Geometry: final body of the model. Coordinates: model frame, mm. Give positions to 0.01 mm unless a question says otherwise; leave off trailing zeros. Order: outer loops, then holes, each group sorted by start corner. A loop starts at its lowest first (then second) coordinate and runs counter-clockwise, first axis right, second up. Notation, with made-up numbers: (22.25, -28) - (70.25, -28) arc R15 ccw to (70.25, -17) - close; hole circle Ø2 at (-28.5, 65). An arc over 180 degrees is marked (long way). Put each result on its own line as item: value. Start each with the question number.
1. Mould query, pull axis X, two halves, no side actions, for faces 1 (the flat face through (30, 30, -8.5)), 2 (the cylindrical face through (48.94, -43.68, -9.01)), 3 (the cylindrical face through (-55.55, -42.594, -8.993)). Classes: pulls with the +X half, pulls with the -X half, needs draft (parallel to the pull), parting line crosses it, or undercut.
2. Section B-B on x = 0. Return the cut outline in (y, z).
3. Section C-C on y = -22. Return the cut outline in (x, z), plus the area to 3 significant figures.
4. Ray query, line 1 along Y through (x, z) = (-6.5, -9.05); line 2 along Y through (x, z) = (41, -8.7); line 3 along Y through (x, z) = (-36.5, -9.1). Return the intervals inside material, ascending. Write a range as from..to.
5. Section D-D on x = 65. Return the cut outline in (y, z), plus the area to 3 significant figures.
6. First-contact query: P1, Ø2.5, axis at x = 42.51, y = 26.32, coming from the -Z side. Flat tip, straight axial feed; report the tip coordinate or a pass-through.
7. Section A-A on y = 0. Return the cut outline in (x, z) (3 decimals), plus the area to 4 significant figures.
from build123d import *

# Parameters (mm, degrees)
SKETCH1_R                                        = 70
CAP_DEPTH                                        = 9.5
SKETCH2_R                                        = 2.125
DOWEL_HOLES_DEPTH                                = 101.801785698
CIRPATTERN1_COUNT                                = 17
SKETCH3_R                                        = 31.05
CENTER_HOLE_DEPTH                                = 15
SKETCH7_R                                        = 40
OUTPUTSHAFT_HOLE_DEPTH                           = 101.124921973
CBORE_FOR_M4_HEX_HEAD_MACHINE_SCREW3_D           = 3.9
CBORE_FOR_M4_HEX_HEAD_MACHINE_SCREW3_DEPTH       = 65
CBORE_FOR_M4_HEX_HEAD_MACHINE_SCREW3_CBORE_D     = 7.5
CBORE_FOR_M4_HEX_HEAD_MACHINE_SCREW3_CBORE_DEPTH = 2.63
CIRPATTERN2_COUNT                                = 8
SKETCH8_R                                        = 37.75
CUT_EXTRUDE4_DEPTH                               = 2
ALLIGNMENT_DEPTH                                 = 100.449736048
ALLIGNMENT_DEPTH_BACK                            = 100.449736048
SKETCH9_W                                        = 157.649556899
SKETCH9_H                                        = 18.162657132


with BuildPart() as part:
    # Sketch1 → Cap (new, symmetric)
    with BuildSketch(Plane.XY):
        Circle(SKETCH1_R)
    extrude(amount=CAP_DEPTH, both=True)

    # Sketch2 → Dowel Holes (cut, through all)
    with BuildSketch(Plane.XY.offset(9.5)):
        with Locations((-50, 0)):
            Circle(SKETCH2_R)
    dowel_holes = extrude(amount=-DOWEL_HOLES_DEPTH, mode=Mode.SUBTRACT)

    # CirPattern1: Dowel Holes ×17 about axis
    cirpattern1_axis = Axis((0, 0, 0), (0, 0, 1))
    for i in range(1, CIRPATTERN1_COUNT):
        add(dowel_holes.rotate(cirpattern1_axis, i * 360 / CIRPATTERN1_COUNT), mode=Mode.SUBTRACT)

    # Sketch3 → Center Hole (cut)
    with BuildSketch(Plane.XY.offset(9.5)):
        Circle(SKETCH3_R)
    extrude(amount=-CENTER_HOLE_DEPTH, mode=Mode.SUBTRACT)

    # Sketch7 → OutputShaft Hole (cut, through all)
    with BuildSketch(Plane.XY.offset(-5.5)):
        Circle(SKETCH7_R)
    extrude(amount=-OUTPUTSHAFT_HOLE_DEPTH, mode=Mode.SUBTRACT)

    # CBORE for M4 Hex Head Machine Screw3
    with Locations(Plane(origin=(0, 0, -9.5), x_dir=(-1, 0, 0), z_dir=(0, 0, -1))):
        with Locations((-65, 0)):
            cbore_for_m4_hex_head_machine_screw3 = CounterBoreHole(CBORE_FOR_M4_HEX_HEAD_MACHINE_SCREW3_D / 2, CBORE_FOR_M4_HEX_HEAD_MACHINE_SCREW3_CBORE_D / 2, CBORE_FOR_M4_HEX_HEAD_MACHINE_SCREW3_CBORE_DEPTH, depth=CBORE_FOR_M4_HEX_HEAD_MACHINE_SCREW3_DEPTH)

    # CirPattern2: CBORE for M4 Hex Head Machine Screw3 ×8 about axis
    cirpattern2_axis = Axis((0, 0, 0), (0, 0, 1))
    for i in range(1, CIRPATTERN2_COUNT):
        add(cbore_for_m4_hex_head_machine_screw3.rotate(cirpattern2_axis, i * 360 / CIRPATTERN2_COUNT), mode=Mode.SUBTRACT)

    # Sketch8 → Cut-Extrude4 (cut)
    with BuildSketch(Plane.XY.offset(9.5)):
        Circle(SKETCH8_R)
    extrude(amount=-CUT_EXTRUDE4_DEPTH, mode=Mode.SUBTRACT)

    # Sketch9 → Allignment (cut, two sides: drawn at the far end of the back side and taken through both)
    with BuildSketch(Plane(origin=(0, 0, 0), x_dir=(1, 0, 0), z_dir=(0, 1, 0)).offset(-ALLIGNMENT_DEPTH_BACK)):
        with Locations((0.351084988, -0.581328566)):
            Rectangle(SKETCH9_W, SKETCH9_H)
    extrude(amount=ALLIGNMENT_DEPTH + ALLIGNMENT_DEPTH_BACK, mode=Mode.SUBTRACT)


solid = part.part
Resolved:
1. face 1: needs draft
1. face 2: undercut
1. face 3: parting line crosses it
2. outline: (-70, -9.5) - (-68.75, -9.5) - (-68.75, -8.5) - (-70, -8.5) - close; (-61.25, -9.5) - (-40, -9.5) - (-40, -8.5) - (-61.25, -8.5) - close; (40, -9.5) - (61.25, -9.5) - (61.25, -8.5) - (40, -8.5) - close; (68.75, -9.5) - (70, -9.5) - (70, -8.5) - (68.75, -8.5) - close
3. outline: (-66.45, -9.5) - (-33.41, -9.5) - (-33.41, -8.5) - (-66.45, -8.5) - close; (33.41, -9.5) - (66.45, -9.5) - (66.45, -8.5) - (33.41, -8.5) - close
3. area: 66.1 mm^2
4. line 1: -69.7..-50.76, -48.81..-39.47, 39.47..48.81, 50.76..69.7
4. line 2: -56.74..-27.82, -24.83..24.83, 27.82..56.74
4. line 3: -59.73..-35.76, -31.61..-16.36, 16.36..31.61, 35.76..59.73
5. outline: (-25.98, -9.5) - (-3.75, -9.5) - (-3.75, -8.5) - (-25.98, -8.5) - close; (3.75, -9.5) - (25.98, -9.5) - (25.98, -8.5) - (3.75, -8.5) - close
5. area: 44.5 mm^2
6. P1: through
7. outline: (-70, -9.5) - (-68.75, -9.5) - (-68.75, -8.5) - (-70, -8.5) - close; (-61.25, -9.5) - (-52.125, -9.5) - (-52.125, -8.5) - (-61.25, -8.5) - close; (-47.875, -9.5) - (-40, -9.5) - (-40, -8.5) - (-47.875, -8.5) - close; (40, -9.5) - (61.25, -9.5) - (61.25, -8.5) - (40, -8.5) - close; (68.75, -9.5) - (70, -9.5) - (70, -8.5) - (68.75, -8.5) - close
7. area: 40.75 mm^2
